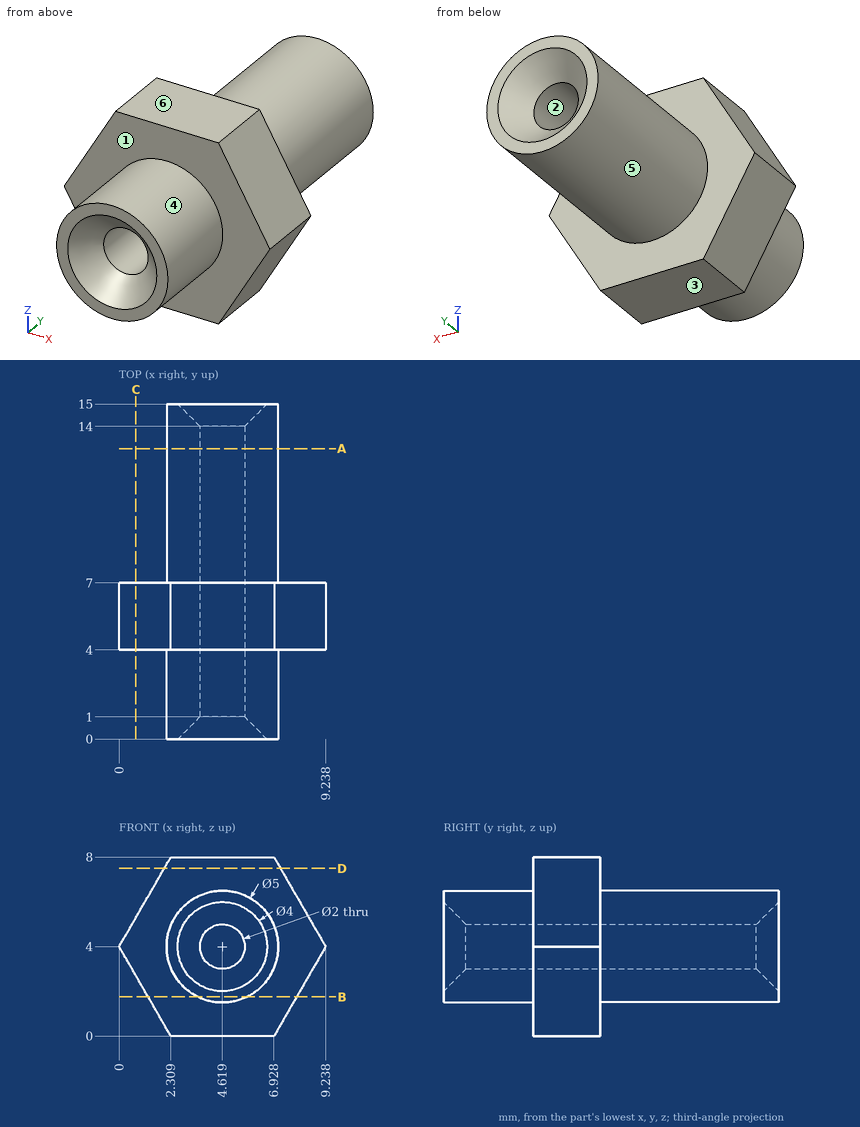
For this review, use the dimensioned drawing (mm, ordinates from the lowest corner) and the shaded views. A direction names the side the tool comes from. Coordinates: 2 decimals unless noted, no trailing zeros. Loops run counter-clockwise (first coordinate to the right, second up) from the corner with the lowest first, then second, coordinate; pieces in that order, holes last. Notation, with made-up numbers: (60, -12.5) -> (115, -12.5) arc R21 ccw to (115, 13.5) -> close; hole circle Ø6 at (86.25, 33). An arc over 180 degrees is marked (long way). Return JSON: item names as keys, results as strings. Group by question number.
(1) Consider section B-B, the plane z = 1.75. Give the boundary of the cut face in (x, y).
(2) Consider section A-A, the plane y = 13. Give the boundary of the cut face in (x, z).
(3) Tool access review of the marked faces 4, 5 and 6: name each direction out of +Z, -Z, +X, -X, +Y, -Y from which nothing blocks a thin tool from reaching the whole face with its end or side.
(4) Consider section D-D, the plane z = 7.5. Give the boundary of the cut face in (x, y), plus the area to 3 significant figures.
(5) Consider section C-C, the plane x = 0.75. Give the boundary of the cut face in (y, z).
(6) For pin 1 Ø1 at (x, z) = (6, 3.5) entering from -Y; pin 2 Ø2 at (x, z) = (2, 1) entering from +Y; pin 3 Ø1.2 at (x, z) = (4.62, 4) entering from -Y; pin 4 Ø1.5 at (x, y) = (5, 10) entering from +Z, all flat-tipped, find the tip position at first contact; note any pin that passes through.
(7) Mouldability with a two-part tool opening along Z and no side actions: class the marked faces 1, 2 and 3 as pulls with the +Z half, pulls with the -Z half, needs draft (parallel to the pull), parting line crosses it, or undercut.
(8) To check wall thickness, follow L1, parallel to X at y = 9.5, z = 4; L2, parallel to Y at x = 2, z = 3.75; L3, parallel to Z at x = 4.25, y = 4.5. State the ranges of each line that lie inside material, in increasing order.
Results below:
{
 "1": {"outline": "(1.3, 4) -> (3.53, 4) -> (3.53, 0) -> (5.71, 0) -> (5.71, 4) -> (7.94, 4) -> (7.94, 7) -> (5.71, 7) -> (5.71, 15) -> (3.53, 15) -> (3.53, 7) -> (1.3, 7) -> close"},
 "2": {"outline": "circle Ø5 at (4.62, 4); hole circle Ø2 at (4.62, 4)"},
 "3": {"face 4": "-Y", "face 5": "+Y", "face 6": "+Z, +X, -X, +Y, -Y"},
 "4": {"outline": "(2.02, 4) -> (7.22, 4) -> (7.22, 7) -> (2.02, 7) -> close", "area": "15.6 mm2"},
 "5": {"outline": "(4, 2.7) -> (7, 2.7) -> (7, 5.3) -> (4, 5.3) -> close"},
 "6": {"pin 1": "stops at y = 0.03", "pin 2": "stops at y = 7", "pin 3": "passes through", "pin 4": "stops at z = 6.5"},
 "7": {"face 1": "needs draft", "face 2": "undercut", "face 3": "pulls with the -Z half"},
 "8": {"L1": "x = 2.12 to 3.62, 5.62 to 7.12", "L2": "y = 4 to 7", "L3": "z = 0 to 3.07, 4.93 to 8"}
}
